Read the model definition and answer for the solid it produces. Units are mm, in the model's axes. A direction names the side the tool comes from. Round coordinates to 2 decimals unless told otherwise and drop trailing zeros. Loops run counter-clockwise (first coordinate to the right, second up) from the corner with the lowest first, then second, coordinate; pieces in that order, holes last. Notation, with made-up numbers: (-2.5, -16.5) - (10.5, -16.5) arc R16 cw to (10.5, -8.5) - close; hole circle Ø1 at (28.25, 35). An arc over 180 degrees is marked (long way). Use CSV: the item, a comma, the result in double quotes. Start each with the question number.
1. Determine the mould class of faces 1 (the cylindrical face through (256.5, -8.57, 0.39)), 2 (the cylindrical face through (8.5, -141.43, 0.39)), 3 (the flat face through (93, -2, 0.8)) for opening direction X: +X half, -X half, draft (parallel to the pull), parting line (faces both ways), or undercut.
2. A tool of negligible diameter and unlimited length cuts with its end or side. For faces 4 (the flat face through (93, -2, 0)), 5 (the cylindrical face through (8.57, -8.5, 0.39)), from which of +Z, -Z, +X, -X, +Y, -Y can it reach the whole face along a straight path? Write none if from no direction.
3. Find section B-B (x = 122). Give the vertices of the cut face in (y, z), and give its area (3 significant figures).
4. Find section C-C (z = 0.55). State how many separate pieces and enclosed holes the cut face has, and give its area (3 significant figures).
5. Consider line 1 along Y through (x, z) = (132.5, 0.65); line 2 along X through (y, z) = (-117.5, 0.3); line 3 along Y through (x, z) = (148, 0.4). Determine where each line is inside the solid, lowest interval first.
6. Find section A-A (y = -55). Give the vertices of the cut face in (x, z).
7. Given pin 1 Ø3.5 at (x, y) = (260, -145) entering from -Z; pin 2 Ø5.5 at (x, y) = (132.5, -145) entering from +Z, each flat-ended and moving along its own axis, determine where each tip first touches the part or whether it passes through.
Autodesk Inventor part; units mm, degrees
ref_plane "YZ Plane" through (0, 0, 0) normal (1, 0, 0) x (0, 1, 0)
ref_plane "XZ Plane" through (0, 0, 0) normal (0, 1, 0) x (-1, 0, 0)
ref_plane "XY Plane" through (0, 0, 0) normal (0, 0, 1) x (1, 0, 0)
sketch "Sketch1" plane through (0, 0, 0) normal (0, 0, 1) x (1, 0, 0)
  line L0 (0, 0) -> (265, 0)
  line L1 (265, 0) -> (265, -150)
  line L2 (265, -150) -> (0, -150)
  line L3 (0, -150) -> (0, 0)
  line L4 (260, -5) -> (5, -5)
  line L5 (5, -5) -> (5, -145)
  line L6 (5, -145) -> (260, -145)
  line L7 (260, -145) -> (260, -5)
  circle A0 centre (5, -5) radius 5
  circle A1 centre (260, -5) radius 5
  circle A2 centre (260, -145) radius 5
  circle A3 centre (5, -145) radius 5
  line L8 (5, -5) -> (5, -75)
  circle A4 centre (5, -75) radius 5
  line L9 (260, -5) -> (260, -75)
  circle A5 centre (260, -75) radius 5
  line L10 (5, -5) -> (132.5, -5)
  circle A6 centre (132.5, -5) radius 5
  line L11 (5, -145) -> (132.5, -145)
  circle A7 centre (132.5, -145) radius 5
  circle A8 centre (5, -5) radius 2.05
  circle A9 centre (5, -75) radius 2.05
  circle A10 centre (5, -145) radius 2.05
  circle A11 centre (132.5, -145) radius 2.05
  circle A12 centre (260, -145) radius 2.05
  circle A13 centre (260, -75) radius 2.05
  circle A14 centre (260, -5) radius 2.05
  circle A15 centre (132.5, -5) radius 2.05
  point P0 (5, -140)
  point P1 (5, -80)
  point P2 (5, -70)
  point P3 (5, -10)
  point P4 (10, -5)
  point P5 (127.5, -5)
  point P6 (137.5, -5)
  point P7 (255, -5)
  point P8 (260, -10)
  point P9 (260, -70)
  point P10 (260, -80)
  point P11 (260, -140)
  point P12 (255, -145)
  point P13 (137.5, -145)
  point P14 (127.5, -145)
  point P15 (10, -145)
  dimension "d0" = 265
  dimension "d1" = 150
  dimension "d2" = 5
  dimension "d3" = 10
  dimension "d4" = 10
  dimension "d5" = 10
  dimension "d6" = 10
  dimension "d7" = 70
  dimension "d8" = 10
  dimension "d9" = 70
  dimension "d10" = 10
  dimension "d11" = 127.5
  dimension "d12" = 10
  dimension "d13" = 127.5
  dimension "d14" = 10
  dimension "d15" = 4.1
  dimension "d16" = 4.1
  dimension "d17" = 4.1
  dimension "d18" = 4.1
  dimension "d19" = 4.1
  dimension "d20" = 4.1
  dimension "d21" = 4.1
  dimension "d22" = 4.1
extrude "Extrusion1" add sketch "Sketch1" along normal blind 0.8 contours L0 A0 L3 | L0 A6 L4 A0 | A0 L4 A8 L5 | A0 L5 A4 L3 | L0 A1 L4 A6 | A6 L4 A15 | A0 L5 A8 L4 | A4 L5 A3 L3 | A4 L5 A9 | L0 L1 A1 | A1 L7 A14 L4 | A6 L4 A15 | A3 L2 L3 | A3 L5 A10 L6 | A4 L5 A9 | L1 A5 L7 A1 | L4 A14 L7 A1 | A3 L6 A10 L5 | A3 L6 A7 L2 | A5 L7 A13 | L1 A2 L7 A5 | A7 L6 A2 L2 | A7 L6 A11 | A2 L6 A12 L7 | L1 L2 A2 | L7 A13 A5 | A7 L6 A11 | L7 A12 L6 A2
properties part number "Empaque"
Filled sheet:
1,face 1,"undercut"
1,face 2,"undercut"
1,face 3,"draft"
2,face 4,"-Z, +X, -X, +Y, -Y"
2,face 5,"+Z, -Z"
3,outline,"(-150, 0) - (-145, 0) - (-145, 0.8) - (-150, 0.8) - close; (-5, 0) - (0, 0) - (0, 0.8) - (-5, 0.8) - close"
3,area,"8.00 mm²"
4,separate pieces,"1"
4,enclosed holes,"9"
4,area,"4,180 mm²"
5,line 1,"y = -150 to -147.05, -142.95 to -140, -10 to -7.05, -2.95 to 0"
5,line 2,"x = 0 to 5, 260 to 265"
5,line 3,"y = -150 to -145, -5 to 0"
6,outline,"(0, 0) - (5, 0) - (5, 0.8) - (0, 0.8) - close; (260, 0) - (265, 0) - (265, 0.8) - (260, 0.8) - close"
7,pin 1,"passes through"
7,pin 2,"stops at z = 0.8"
